The drawing under review shows one solid part. Ordinate dimensions are in mm from its lowest x, y, z. Give positions to 0.01 mm unless a question says otherwise; leave off trailing zeros. Loops run counter-clockwise (first coordinate to the right, second up) from the corner with the lowest first, then second, coordinate; pieces in that order, holes last. Notation, with made-up numbers: M -40,-32 L -1,-32 A19 ccw -1,3 Z; hole C 22,-15.5 d7. An arc over 180 degrees is marked long. Answer as CSV lines item,"result".
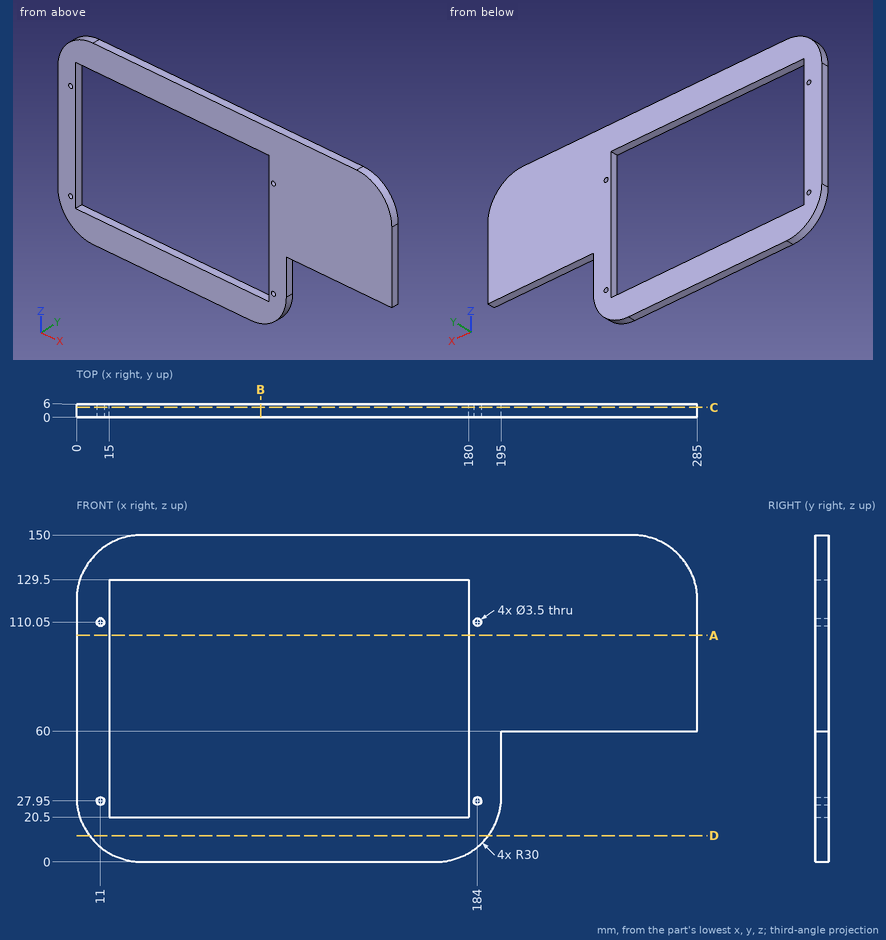
1. To check wall thickness, follow L1, parallel to X at y = 2.5, z = 110; L2, parallel to Z at x = 84, y = 0.55; L3, parallel to X at y = 3.6, z = 27.95. State the ranges of each line that lie inside material, in increasing order. Write a range as [from, to].
Answer block:
L1,"[0, 9.25], [12.75, 15], [180, 182.25], [185.75, 285]"
L2,"[0, 20.5], [129.5, 150]"
L3,"[0.07, 9.25], [12.75, 15], [180, 182.25], [185.75, 194.93]"
2. We need section B-B, the plane x = 84.5. Write out the cut boundary in (y, z), plus the area to 3 significant figures.
Answer block:
outline,"M 0,0 L 6,0 L 6,20.5 L 0,20.5 Z; M 0,129.5 L 6,129.5 L 6,150 L 0,150 Z"
area,"246 mm²"
3. We need section A-A, the plane z = 104. Write out the cut boundary in (x, y).
Answer block:
outline,"M 0,0 L 15,0 L 15,6 L 0,6 Z; M 180,0 L 285,0 L 285,6 L 180,6 Z"
4. For P1, Ø5, axis at x = 170, z = 128.5, coming from the -Y side; P2, Ø3, axis at y = 4.5, z = 45.5, coming from the +X side; P3, Ø3, axis at x = 184, z = 27.95, coming from the -Y side; P4, Ø2, axis at y = 4, z = 133, coming from the +X side, all flat-tipped, find the tip position at first contact; note any pin that passes through.
Answer block:
P1,"y = 0"
P2,"x = 195"
P3,"through"
P4,"x = 282.5"
5. We need section C-C, the plane y = 4.5. Write out the cut boundary in (x, z).
Answer block:
outline,"M 0,30 A30 ccw 30,0 L 165,0 A30 ccw 195,30 L 195,60 L 285,60 L 285,120 A30 ccw 255,150 L 30,150 A30 ccw 0,120 Z; hole C 11,27.95 d3.5; hole C 11,110.05 d3.5; hole M 15,20.5 L 180,20.5 L 180,129.5 L 15,129.5 Z; hole C 184,27.95 d3.5; hole C 184,110.05 d3.5"
6. We need section D-D, the plane z = 12. Write out the cut boundary in (x, y).
Answer block:
outline,"M 6,0 L 189,0 L 189,6 L 6,6 Z"
